Part model, mm, in its own coordinate system. Coordinates: 2 decimals unless noted, no trailing zeros. Use a Markdown table: item, result. Add a question column.
Q1. Mould opens along X. For faces 1 (the cylindrical face through (-15.727, -28.09, 2.571)), 2 (the flat face through (-33, -19, 0)), 3 (the cylindrical face through (-34.654, -28.061, 12.774)) say: released by +X, released by -X, zero draft, split by the parting line, or undercut.
Q2. Wall check: L1, parallel to X at y = -28.5, z = 2; L2, parallel to Y at x = -18, z = 10.25; L3, parallel to X at y = -15.25, z = 16.5. Give the ranges that are in metal, low to high. Write a range as from..to.
Q3. Pin check, flat tips, straight feed: pin 1 Ø1 at (x, z) = (-15.5, 9) entering from -Y; pin 2 Ø4 at (x, z) = (-36.5, 4.5) entering from -Y; pin 3 Ø1.5 at (y, z) = (-18.5, 12) entering from -X. Stop position of each tip, or through.
from build123d import *

# Parameters (mm, degrees)
F4_R     = 1.5875
F5_DEPTH = 3.175
F6_R     = 0.254


with BuildPart() as f3:
    # F2 (on offset) → F3 section 0
    with BuildSketch(Plane.XY.offset(19.05)):
        Polygon((-47.3329591776, -20.2521206051), (-47.3329591776, -26.6021206051), (-18.5506157587, -26.6021206051), (-18.5506157587, -20.2521206051), (-32.9417874681, -12.1605029158), align=None)
    # F0 (on Top) → F3 section 1
    with BuildSketch(Plane.XY):
        Polygon((-55.9284321933, -20.3077479873), (-55.9284321933, -26.6577479873), (-10.2084321933, -26.6577479873), (-10.2084321933, -20.3077479873), (-33.0684321933, -9.2361446707), align=None)
    loft()

    # F4 (on face) → F5 (join)
    with BuildSketch(Plane(origin=(0, -26.6575206833, 0.0778418945), x_dir=(1, 0, 0), z_dir=(0, -0.9999957366, 0.0029200601))):
        with Locations((-48.9434321933, 3.0971577737)):
            Circle(F4_R)
        with Locations((-33.0684321933, 12.6221577737)):
            Circle(F4_R)
        with Locations((-17.1934321933, 3.0971577737)):
            Circle(F4_R)
    extrude(amount=F5_DEPTH)

    # F6
    f6_edges = [f3.edges().sort_by_distance(p)[0] for p in [
        (-50.530932, -29.823463, 3.184258),
        (-34.655932, -29.79565, 12.709217),
        (-18.780932, -29.823463, 3.184258),
    ]]
    fillet(f6_edges, radius=F6_R)


solid = f3.part
Recorded:
| question | item | result |
|---|---|---|
| 1 | face 1 | undercut |
| 1 | face 2 | zero draft |
| 1 | face 3 | split by the parting line |
| 2 | L1 | -50..-47.88, -18.25..-16.13 |
| 2 | L2 | -26.63..-18.57 |
| 2 | L3 | -39.32..-26.59 |
| 3 | pin 1 | y = -26.63 |
| 3 | pin 2 | y = -26.65 |
| 3 | pin 3 | x = -48.6 |
